Could you check a few things on this drawing? It's one solid part, dimensions in mm from its lowest x, y, z. Give positions to 0.01 mm unless a question says otherwise; leave off trailing zeros. Order: outer loops, then holes, each group sorted by start corner. A loop starts at its lowest first (then second) coordinate and runs counter-clockwise, first axis right, second up. Notation, with made-up numbers: M -16.5,10 L 7.5,10 A23 ccw 7.5,36 Z; hole C 45,72.25 d2. An arc over 180 degrees is marked long. One line per item, written item: value. Start each with the question number.
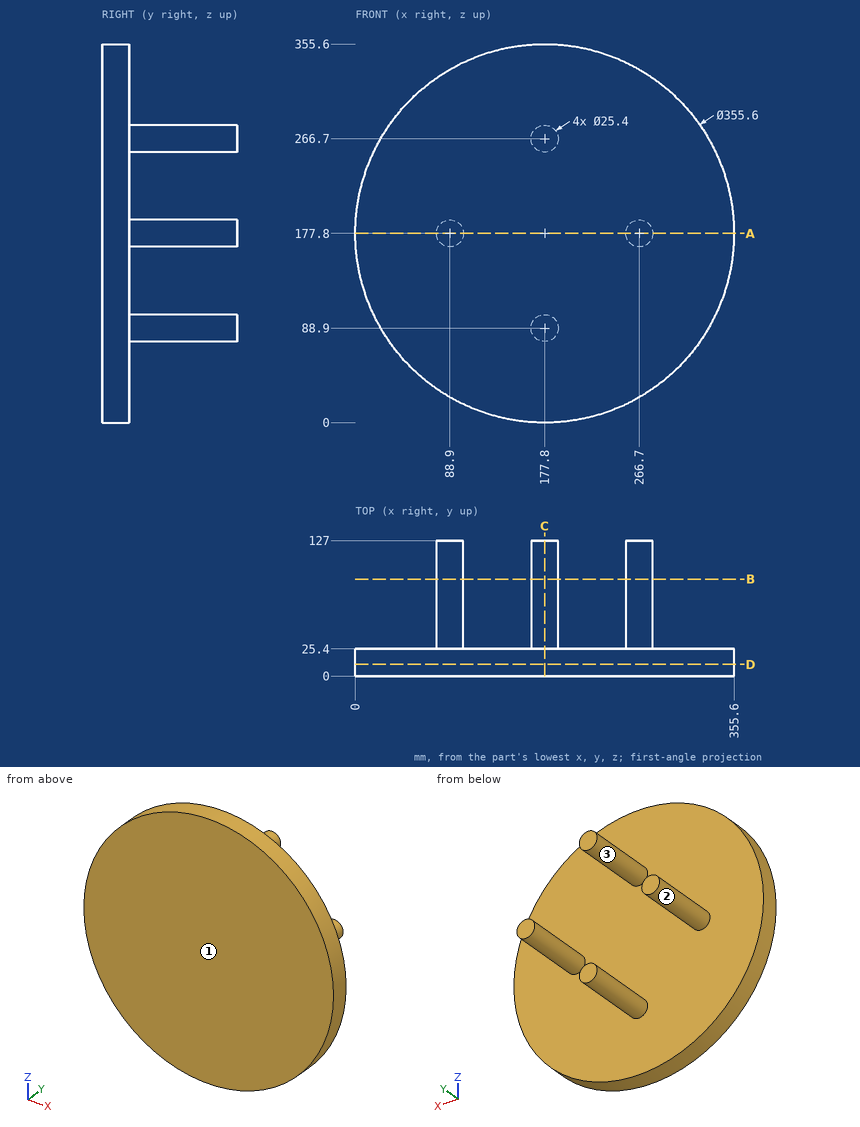
Item 1: I want a section at C-C on x = 177.8. Write out the boundary of the cut face in (y, z).
Item 2: I want a section at A-A on z = 177.8. Write out the boundary of the cut face in (x, y), plus the area to 3 significant figures.
Item 3: We'd pull the mould along X, two halves only. Please class the marked faces 1, 2 and 3: +X half, -X half, draft (parallel to the pull), parting line (faces both ways), or undercut.
Item 4: I want a section at D-D on y = 11. Write out the boundary of the cut face in (x, z), plus the area to 3 significant figures.
Item 5: Please list where these lines run through material, in increasing order: probe 1 along Y at (x, z) = (179.5, 173); probe 2 along X at (y, z) = (69, 184.5); probe 3 along X at (y, z) = (23, 134). Write a range as [from, to].
Item 6: I want a section at B-B on y = 91. Write out the boundary of the cut face in (x, z).
Item 7: Will these pins go through, and if not, where does the flat tip stop? P1, Ø1, axis at x = 286.5, z = 119, coming from the +Y side; P2, Ø3, axis at y = 83.5, z = 183, coming from the +X side; P3, Ø12, axis at y = 102.5, z = 271, coming from the -X side.
Answer below:
1. outline: M 0,0 L 25.4,0 L 25.4,76.2 L 127,76.2 L 127,101.6 L 25.4,101.6 L 25.4,254 L 127,254 L 127,279.4 L 25.4,279.4 L 25.4,355.6 L 0,355.6 Z
2. outline: M 0,0 L 355.6,0 L 355.6,25.4 L 279.4,25.4 L 279.4,127 L 254,127 L 254,25.4 L 101.6,25.4 L 101.6,127 L 76.2,127 L 76.2,25.4 L 0,25.4 Z
2. area: 14,200 mm²
3. face 1: draft
3. face 2: undercut
3. face 3: parting line
4. outline: C 177.8,177.8 d355.6
4. area: 99,300 mm²
5. probe 1: y = [0, 25.4]
5. probe 2: x = [78.11, 99.69], [255.91, 277.49]
5. probe 3: x = [5.48, 350.12]
6. outline: C 88.9,177.8 d25.4; C 177.8,88.9 d25.4; C 177.8,266.7 d25.4; C 266.7,177.8 d25.4
7. P1: stops at y = 25.4
7. P2: stops at x = 278.85
7. P3: stops at x = 165.1
